Source: CAD feature listing. Evaluate the final solid. Frame: model axes, mm. A direction names the side the tool comes from. Give positions to 0.01 mm unless a question says otherwise; leave off trailing zeros. Order: outer loops, then holes, each group sorted by start corner. A loop starts at its lowest first (then second) coordinate and runs counter-clockwise, first axis right, second up.
```python
from build123d import *

# Parameters (mm, degrees)
SKETCH_1_R                = 17.63
SKETCH_1_R_2              = 14.34
EXTRUDE_1_DEPTH           = 16.05
EXTRUDE_1_2_DEPTH         = 9.77
EXTRUDE_1_2_DEPTH_BACK    = 3
SKETCH_2_W                = 16
SKETCH_2_H                = 16.05
SKETCH_3_W                = 3.41
SKETCH_3_H                = 16
CUT_EXTRUDE_1_DEPTH       = 37.411121927
SKETCH_4_R                = 1.91
CUT_EXTRUDE_2_DEPTH       = 39.675463798
EXTRUDE_2_DEPTH           = 4
EXTRUDE_2_DEPTH_BACK      = 2.77
SKETCH_5_W                = 12.19
SKETCH_5_H                = 8.263625949
SKETCH_6_W                = 12.19
SKETCH_6_H                = 6.77
EXTRUDE_3_DEPTH           = 63
SKETCH_8_W                = 12.19
SKETCH_8_H                = 6.77
EXTRUDE_4_DEPTH           = 0.16
EXTRUDE_5_DEPTH           = 3.16
EXTRUDE_5_DEPTH_BACK      = 10
SKETCH_12_W               = 16
SKETCH_12_H               = 16.05
SKETCH_13_W               = 1.21
SKETCH_13_H               = 16
CUT_EXTRUDE_3_DEPTH       = 73.543164889
SKETCH_14_R               = 1.91
CUT_EXTRUDE_4_DEPTH       = 90.07387176
SKETCH_15_R               = 4.05
CUT_EXTRUDE_5_DEPTH       = 24
SKETCH_16_W               = 56.400519221
SKETCH_16_H               = 19.935010357
CUT_EXTRUDE_6_DEPTH       = 73.088971918
SKETCH_17_W               = 12.19
SKETCH_17_H               = 71.423625949
EXTRUDE_7_DEPTH           = 25
SKETCH_18_W               = 26.793372528
SKETCH_18_H               = 63.398625949
CUT_EXTRUDE_7_DEPTH       = 25
SKETCH_19_R               = 4
CUT_EXTRUDE_8_DEPTH       = 24
CUT_EXTRUDE_9_DEPTH       = 29
EXTRUDE_9_DEPTH           = 2
FILLET_1_R                = 10
SKETCH_24_W               = 12.19
SKETCH_24_H               = 5
EXTRUDE_10_DEPTH          = 27
SKETCH_27_W               = 12.19
SKETCH_27_H               = 10.03
EXTRUDE_11_DEPTH          = 20.23
CUT_EXTRUDE_10_DEPTH      = 45.23
CUT_EXTRUDE_10_DEPTH_BACK = 8
SKETCH_21_W               = 8
SKETCH_21_H               = 16
SKETCH_25_W               = 20.230462415
SKETCH_25_H               = 10.025
CUT_EXTRUDE_12_DEPTH      = 20.23
SKETCH_31_W               = 8
SKETCH_31_H               = 2.03
EXTRUDE_13_DEPTH          = 16.23
EXTRUDE_17_DEPTH          = 10


with BuildPart() as part:
    # 草圖1 → Extrude 1 (new body)
    with BuildSketch(Plane(origin=(0, 0, 0), x_dir=(1, 0, 0), z_dir=(0, 1, 0))):
        Circle(SKETCH_1_R)
        Circle(SKETCH_1_R_2, mode=Mode.SUBTRACT)
    extrude(amount=EXTRUDE_1_DEPTH)

    # 草圖2 → Extrude 1 2 (add, two sides: drawn at the far end of the back side and taken through both)
    with BuildSketch(Plane(origin=(17.75, 0, 0), x_dir=(0, 0, -1), z_dir=(1, 0, 0)).offset(-EXTRUDE_1_2_DEPTH_BACK)):
        with Locations((0, 8.025)):
            Rectangle(SKETCH_2_W, SKETCH_2_H)
    extrude(amount=EXTRUDE_1_2_DEPTH + EXTRUDE_1_2_DEPTH_BACK)

    # 草圖3 → 除料-伸長1 (cut, through all)
    with BuildSketch(Plane(origin=(0, 16.05, 0), x_dir=(1, 0, 0), z_dir=(0, 1, 0))):
        with Locations((25.815, 0)):
            Rectangle(SKETCH_3_W, SKETCH_3_H)
    extrude(amount=-CUT_EXTRUDE_1_DEPTH, mode=Mode.SUBTRACT)

    # 草圖4 → 除料-伸長2 (cut, through all)
    with BuildSketch(Plane.XY.offset(8)):
        with Locations((19.910203689, 8.025)):
            Circle(SKETCH_4_R)
    extrude(amount=-CUT_EXTRUDE_2_DEPTH, mode=Mode.SUBTRACT)

    # 草圖5 → 填料-伸長2 (add, two sides: drawn at the far end of the back side and taken through both)
    with BuildSketch(Plane.XY.offset(17.75).offset(-EXTRUDE_2_DEPTH_BACK)):
        with Locations((0, 12.156812974)):
            Rectangle(SKETCH_5_W, SKETCH_5_H)
    extrude(amount=EXTRUDE_2_DEPTH + EXTRUDE_2_DEPTH_BACK)

    # 草圖6 → 填料-伸長3 (add)
    with BuildSketch(Plane(origin=(0, 16.288625949, 0), x_dir=(1, 0, 0), z_dir=(0, 1, 0))):
        with Locations((0, -18.365)):
            Rectangle(SKETCH_6_W, SKETCH_6_H)
    extrude(amount=EXTRUDE_3_DEPTH)

    # 草圖8 → 填料-伸長4 (add)
    with BuildSketch(Plane(origin=(0, 79.288625949, 0), x_dir=(1, 0, 0), z_dir=(0, 1, 0))):
        with Locations((0, -18.365)):
            Rectangle(SKETCH_8_W, SKETCH_8_H)
    extrude(amount=EXTRUDE_4_DEPTH)

    # 草圖12 → 填料-伸長5 (add, two sides: drawn at the far end of the back side and taken through both)
    with BuildSketch(Plane(origin=(-17.75, 0, 0), x_dir=(0, 0, -1), z_dir=(1, 0, 0)).offset(-EXTRUDE_5_DEPTH_BACK)):
        with Locations((0.543544944, 8.025)):
            Rectangle(SKETCH_12_W, SKETCH_12_H)
    extrude(amount=EXTRUDE_5_DEPTH + EXTRUDE_5_DEPTH_BACK)

    # 草圖13 → 除料-伸長3 (cut, through all)
    with BuildSketch(Plane(origin=(0, 16.05, 0), x_dir=(1, 0, 0), z_dir=(0, 1, 0))):
        with Locations((-27.145, 0.543544944)):
            Rectangle(SKETCH_13_W, SKETCH_13_H)
    extrude(amount=-CUT_EXTRUDE_3_DEPTH, mode=Mode.SUBTRACT)

    # 草圖14 → 除料-伸長4 (cut, through all)
    with BuildSketch(Plane(origin=(0, 0, -8.543544944), x_dir=(-1, 0, 0), z_dir=(0, 0, -1))):
        with Locations(Location((20.980783679, 8.025, 0), (0, 0, 90))):
            Circle(SKETCH_14_R)
    extrude(amount=-CUT_EXTRUDE_4_DEPTH, mode=Mode.SUBTRACT)

    # 草圖15 → 除料-伸長5 (cut)
    with BuildSketch(Plane(origin=(0, 79.448625949, 0), x_dir=(1, 0, 0), z_dir=(0, 1, 0))):
        with Locations((0, -14.98)):
            Circle(SKETCH_15_R)
    extrude(amount=-CUT_EXTRUDE_5_DEPTH, mode=Mode.SUBTRACT)

    # 草圖16 → 除料-伸長6 (cut, through all)
    with BuildSketch(Plane(origin=(0, 16.05, 0), x_dir=(1, 0, 0), z_dir=(0, 1, 0))):
        with Locations((-4.090259611, 9.967505179)):
            Rectangle(SKETCH_16_W, SKETCH_16_H)
    extrude(amount=-CUT_EXTRUDE_6_DEPTH, mode=Mode.SUBTRACT)

    # 草圖17 → 填料-伸長7 (add)
    with BuildSketch(Plane.XY.offset(21.75)):
        with Locations((0, 43.736812975)):
            Rectangle(SKETCH_17_W, SKETCH_17_H)
    extrude(amount=EXTRUDE_7_DEPTH)

    # 草圖18 → 除料-伸長7 (cut)
    with BuildSketch(Plane.ZY.offset(6.095)):
        with Locations((28.376686264, 47.749312975)):
            Rectangle(SKETCH_18_W, SKETCH_18_H)
    extrude(amount=-CUT_EXTRUDE_7_DEPTH, mode=Mode.SUBTRACT)

    # 草圖19 → 除料-伸長8 (cut)
    with BuildSketch(Plane(origin=(0, 79.448625949, 0), x_dir=(1, 0, 0), z_dir=(0, 1, 0))):
        with Locations((0, -41.773372528)):
            Circle(SKETCH_19_R)
    extrude(amount=-CUT_EXTRUDE_8_DEPTH, mode=Mode.SUBTRACT)

    # 草圖20 → 除料-伸長9 (cut)
    with BuildSketch(Plane(origin=(6.095, 0, 0), x_dir=(0, 0, -1), z_dir=(1, 0, 0))):
        Polygon((-41.773372528, 16.05), (-41.773372528, 8.025), (-46.75, 8.025), (-46.75, 79.448625949), (-41.773372528, 79.448625949), align=None)
    extrude(amount=-CUT_EXTRUDE_9_DEPTH, mode=Mode.SUBTRACT)

    # 草圖23 → 填料-伸長9 (add)
    with BuildSketch(Plane.XZ.offset(-8.025)):
        Polygon((-6.095, 41.773372528), (-6.095, 17.75), (6.13829314, 17.75), (6.095, 41.773372528), align=None)
    extrude(amount=EXTRUDE_9_DEPTH)

    # 圓角1
    # the kernel refuses this fillet: 10 mm, written as the material it takes off along each edge
    with BuildSketch(Plane(origin=(-21.095, 6.025, 17.75), x_dir=(0, 1, 0), z_dir=(1, 0, 0))) as fillet_1_piece_1:
        with BuildLine():
            CenterArc((10, 6), FILLET_1_R, 180, 36.869897646)
            Line((0, 6), (0, 0))
            Line((0, 0), (2, 0))
        make_face()
    extrude(amount=42.23329314, mode=Mode.SUBTRACT)

    # 草圖24 → 填料-伸長10 (add)
    with BuildSketch(Plane(origin=(0, 16.05, 0), x_dir=(1, 0, 0), z_dir=(0, 1, 0))):
        with Locations((0, -19.042910113)):
            Rectangle(SKETCH_24_W, SKETCH_24_H)
    extrude(amount=EXTRUDE_10_DEPTH)

    # 草圖27 → 填料-伸長11 (add)
    with BuildSketch(Plane.XY.offset(21.542910113)):
        with Locations((0, 38.035)):
            Rectangle(SKETCH_27_W, SKETCH_27_H)
    extrude(amount=EXTRUDE_11_DEPTH)

    # 草圖21 → 除料-伸長10 (cut, two sides: drawn at the far end of the back side and taken through both)
    with BuildSketch(Plane(origin=(0, 16.05, 0), x_dir=(1, 0, 0), z_dir=(0, 1, 0)).offset(-CUT_EXTRUDE_10_DEPTH_BACK)):
        with Locations((0, -28)):
            Rectangle(SKETCH_21_W, SKETCH_21_H)
    extrude(amount=CUT_EXTRUDE_10_DEPTH + CUT_EXTRUDE_10_DEPTH_BACK, mode=Mode.SUBTRACT)

    # 草圖25 → 除料-伸長12 (cut)
    with BuildSketch(Plane.ZY.offset(6.095)):
        with Locations((31.658141321, 11.0375)):
            Rectangle(SKETCH_25_W, SKETCH_25_H)
    extrude(amount=-CUT_EXTRUDE_12_DEPTH, mode=Mode.SUBTRACT)

    # 草圖31 → 填料-伸長13 (add)
    with BuildSketch(Plane(origin=(0, 0, 36), x_dir=(-1, 0, 0), z_dir=(0, 0, -1))):
        with Locations((0, 34.035)):
            Rectangle(SKETCH_31_W, SKETCH_31_H)
    extrude(amount=EXTRUDE_13_DEPTH)

    # 草圖33 → 填料-伸長17 (add)
    with BuildSketch(Plane.XY.offset(21.542910113)):
        Polygon((-6.095, 33.02), (-4, 33.02), (-4, 8.05), (4, 8.05), (4, 33.02), (6.095, 33.02), (6.131457839, 6.271602939), (-6.095, 6.271602939), align=None)
    extrude(amount=EXTRUDE_17_DEPTH)


solid = part.part
```
1) Section query B-B, the plane z = 27. Return the cut outline in (x, y) (3 decimals).
Report:
outline: (-6.095, 6.272) - (6.131, 6.272) - (6.095, 33.02) - (6.095, 43.05) - (4, 43.05) - (4, 35.05) - (-4, 35.05) - (-4, 43.05) - (-6.095, 43.05) - close; hole (-4, 8.05) - (4, 8.05) - (4, 33.02) - (-4, 33.02) - close
2) Reachability of faces 1 (the flat face through (-6.095, 28, 26)), 2 (the flat face through (0, 39, 20)), 3 (the flat face through (-4, 21, 26)), 4 (the flat face through (0, 6.272, 26)) from +Z, -Z, +X, -X, +Y, -Y: full face, straight path, thin tool, end or side. Return the list, or none.
Report:
face 1: +Z, -X, +Y, -Y
face 2: +Y
face 3: +Z
face 4: +Z, +X, -X, -Y
3) Pin query (flat end, axial travel): pin 1 (9 mm diameter, centred on y = 40, z = 24, fed in from +X) (3 decimals); pin 2 (2.5 mm diameter, centred on x = 0, z = 30.5, fed in from +Y); pin 3 (4 mm diameter, centred on x = -9, y = 27.5, fed in from +Z); pin 4 (12 mm diameter, centred on x = -13, z = 14.5, fed in from +Y). Return the tip coordinate at first contact, or that it passes through.
Report:
pin 1: stops at x = 6.095
pin 2: stops at y = 35.05
pin 3: passes through
pin 4: stops at y = 16.05
4) Section query C-C, the plane x = 0. Return the cut outline in (y, z) (3 decimals).
Report:
outline: (0, 14.34) - (16.05, 14.34) - (16.05, 16.543) - (43.05, 16.543) - (43.05, 20) - (35.05, 20) - (35.05, 36) - (43.05, 36) - (43.05, 41.773) - (33.02, 41.773) - (33.02, 20) - (8.05, 20) - (8.05, 31.543) - (6.272, 31.543) - (6.272, 21.543) arc R10 ccw to (8.025, 17.75) - (8.025, 17.63) - (0, 17.63) - close
5) Section query D-D, the plane z = 33.5. Return the cut outline in (x, y) (3 decimals).
Report:
outline: (-6.095, 33.02) - (6.095, 33.02) - (6.095, 43.05) - (4, 43.05) - (4, 35.05) - (-4, 35.05) - (-4, 43.05) - (-6.095, 43.05) - close
6) Draft query along Y for faces 5 (the flat face through (-4, 39, 28)), 6 (the cylindrical face through (-0.064, 6.936, 19.581)), 7 (the flat face through (0, 8.05, 26)). Return one class per face: +Y half, -Y half, draft (parallel to the pull), parting line (faces both ways), or undercut.
Report:
face 5: draft
face 6: -Y half
face 7: undercut
7) Material intervals for L1, parallel to X at y = 18, z = 21 (3 decimals); L2, parallel to Y at x = -3.5, z = 24.5; L3, parallel to X at y = 8.5, z = 5, sorted ascending.
Report:
L1: x = -6.095 to -4, 4 to 6.095
L2: y = 6.27 to 8.05, 33.02 to 35.05
L3: x = -26.54 to -22.83, -19.13 to -13.44, 13.44 to 18.06, 21.76 to 24.11
8) Section query A-A, the plane z = 5.5. Return the cut outline in (x, y) (3 decimals), and give its area (3 significant figures).
Report:
outline: (-26.54, 0) - (-13.243, 0) - (-13.243, 16.05) - (-26.54, 16.05) - close; (13.243, 0) - (24.11, 0) - (24.11, 16.05) - (13.243, 16.05) - close; hole circle Ø3.82 at (-20.981, 8.025); hole circle Ø3.82 at (19.91, 8.025)
area: 365 mm2
